from build123d import *

# Parameters (mm, degrees)
BOSS_EXTRU_1_DEPTH      = 18
ENL_V_MAT_EXTRU_1_REACH = 82.979
ESQUISSE4_W             = 11
ESQUISSE4_H             = 27
ENL_V_MAT_EXTRU_2_DEPTH = 11
D_GAGEMENT_M31_D        = 3.4
ENL_V_MAT_EXTRU_3_DEPTH = 8.4
ESQUISSE10_R            = 0.9
ENL_V_MAT_EXTRU_4_DEPTH = 4
ENL_V_MAT_EXTRU_5_DEPTH = 5
CONG_1_R                = 2
CONG_2_R                = 8
ENL_V_START             = -1.6
ESQUISSE13_R            = 1.5
ENL_V_MAT_EXTRU_6_DEPTH = 78.3514199


with BuildPart() as part:
    # Esquisse1 → Boss.-Extru.1 (new body)
    with BuildSketch(Plane(origin=(0, 0, 0), x_dir=(0, 0, -1), z_dir=(1, 0, 0))):
        Polygon((-37.5, 64.951905284), (-40.964101615, 62.951905284), (-24.964101615, 35.239092363), (-45.309401077, 0), (0, 0), (-2.309401077, 4), (-8.082903769, 4), (-23.232050808, 30.239092363), (-20.345299462, 35.239092363), align=None)
    extrude(amount=BOSS_EXTRU_1_DEPTH)

    # Esquisse4 → Enlèv. mat.-Extru.1 (cut, up to next)
    with BuildSketch(Plane(origin=(0, -2, 3.464101615), x_dir=(1, 0, 0), z_dir=(0, -0.5000000000000047, 0.8660254037844359)), mode=Mode.PRIVATE) as enl_v_mat_extru_1_sk1:
        with Locations((12.5, 61.5)):
            Rectangle(ESQUISSE4_W, ESQUISSE4_H)
    enl_v_mat_extru_1_tool1 = extrude(enl_v_mat_extru_1_sk1.sketch, amount=-ENL_V_MAT_EXTRU_1_REACH, mode=Mode.PRIVATE) & part.part
    add(enl_v_mat_extru_1_tool1.solids().sort_by_distance((12.5, 51.260562, 34.214102))[0], mode=Mode.SUBTRACT)

    # Esquisse6 → Enlèv. mat.-Extru.2 (cut)
    with BuildSketch(Plane(origin=(18, 0, 0), x_dir=(0, 0, -1), z_dir=(1, 0, 0))):
        Polygon((0, 0), (-2.309401077, 4), (-8.082903769, 4), (-5.773502692, 0), align=None)
    extrude(amount=-ENL_V_MAT_EXTRU_2_DEPTH, mode=Mode.SUBTRACT)

    # Dégagement M31 (through all)
    with Locations(Plane(origin=(0, 0, 0), x_dir=(-1, 0, 0), z_dir=(0, 0.5000000000000047, -0.866025403784436))):
        with Locations((-3.5, 71.2), (-3.5, 46)):
            Hole(D_GAGEMENT_M31_D / 2)

    # Esquisse9 → Enlèv. mat.-Extru.3 (cut)
    with BuildSketch(Plane.ZY):
        with BuildLine():
            Line((19.441451884, 15.2), (20.441451884, 16.2))
            Line((20.441451884, 16.2), (30.641451884, 16.2))
            Line((30.641451884, 16.2), (31.641451884, 15.2))
            Line((31.641451884, 15.2), (31.641451884, 13.4))
            ThreePointArc((31.641451884, 13.4), (32.541451884, 12.5), (31.641451884, 11.6))
            Line((31.641451884, 11.6), (31.641451884, 8.6))
            ThreePointArc((31.641451884, 8.6), (32.541451884, 7.7), (31.641451884, 6.8))
            Line((31.641451884, 6.8), (31.641451884, 5))
            Line((31.641451884, 5), (30.641451884, 4))
            Line((30.641451884, 4), (20.441451884, 4))
            Line((20.441451884, 4), (19.441451884, 5))
            Line((19.441451884, 5), (19.441451884, 6.8))
            ThreePointArc((19.441451884, 6.8), (18.541451884, 7.7), (19.441451884, 8.6))
            Line((19.441451884, 8.6), (19.441451884, 11.6))
            ThreePointArc((19.441451884, 11.6), (18.541451884, 12.5), (19.441451884, 13.4))
            Line((19.441451884, 13.4), (19.441451884, 15.2))
        make_face()
    extrude(amount=-ENL_V_MAT_EXTRU_3_DEPTH, mode=Mode.SUBTRACT)

    # Esquisse10 → Enlèv. mat.-Extru.4 (cut)
    with BuildSketch(Plane.ZY.offset(-8.4)):
        with Locations((19.441451884, 12.5)):
            Circle(ESQUISSE10_R)
        with Locations((19.441451884, 7.7)):
            Circle(ESQUISSE10_R)
        with Locations((31.641451884, 12.5)):
            Circle(ESQUISSE10_R)
        with Locations((31.641451884, 7.7)):
            Circle(ESQUISSE10_R)
    extrude(amount=-ENL_V_MAT_EXTRU_4_DEPTH, mode=Mode.SUBTRACT)

    # Esquisse11 → Enlèv. mat.-Extru.5 (cut)
    with BuildSketch(Plane.ZY):
        Polygon((25.541451884, 26.239092363), (12.701705922, 4), (38.381197846, 4), align=None)
    extrude(amount=-ENL_V_MAT_EXTRU_5_DEPTH, mode=Mode.SUBTRACT)

    # Congé1
    cong_1_edges = [part.edges().sort_by_distance(p)[0] for p in [
        (0, 63.951905284, 39.232050808),
        (2.5, 4, 38.381197846),
        (2.5, 26.239092363, 25.541451884),
        (2.5, 4, 12.701705922),
        (9, 0, 45.309401077),
        (9, 35.239092363, 24.964101615),
        (9, 35.239092363, 20.345299462),
        (9, 30.239092363, 23.232050808),
        (18, 40.569219382, 25.732050808),
        (7, 63.951905284, 39.232050808),
        (3.5, 0, 0),
        (3.5, 4, 8.082903769),
        (3.5, 4, 2.309401077),
        (12.5, 0, 5.773502692),
    ]]
    fillet(cong_1_edges, radius=CONG_1_R - 0.0001)  # a hair under: the kernel refuses the full size

    # Congé2
    cong_2_edges = [part.edges().sort_by_distance(p)[0] for p in [
        (7, 40.569219382, 25.732050808),
    ]]
    fillet(cong_2_edges, radius=CONG_2_R)

    # Esquisse13 → Enlèv. mat.-Extru.6 (cut, through all)
    with BuildSketch(Plane.ZY.offset(-8.4).offset(ENL_V_START)):
        with Locations((19.441451884, 12.5)):
            Circle(ESQUISSE13_R)
        with Locations((19.441451884, 7.7)):
            Circle(ESQUISSE13_R)
    extrude(amount=-ENL_V_MAT_EXTRU_6_DEPTH, mode=Mode.SUBTRACT)


solid = part.part
Read the model definition and answer for the solid it produces. Units are mm, in the model's axes. A direction names the side the tool comes from. Give positions to 0.01 mm unless a question says otherwise; leave off trailing zeros. Write each loop counter-clockwise with the first axis right and the second up, starting at its lowest first coordinate (ties: lowest second). Pieces come first, ordered by that corner, then holes. Notation, with made-up numbers: (-36, -40) - (-21, -40) arc R13 cw to (-21, -21) - close; hole circle Ø8 at (12.25, 18). An arc over 180 degrees is marked (long way). Answer in a Markdown table with one row per item. Add a question column.
Item 1: A tool of negligible diameter and unlimited length cuts with its end or side. For faces 1 (the face through (8.87, 32.72, 21.8)), 2 (the face through (6.87, 47.2, 27.25)), 3 (the face through (3, 4, 25)), 4 (the face through (9.28, 42.67, 26.91)), 5 (the face through (13.94, 7.13, 20.83)), from which of +Z, -Z, +X, -X, +Y, -Y can it reach the whole face along a straight path? Write none if from no direction.
Item 2: Section B-B, the plane z = 33.5 is taken. Write down the section's boundary in (x, y), and give its area (3 significant figures).
Item 3: Determine the mould class of faces 6 (the face through (7, 2, 5)), 7 (the face through (2.54, 24.24, 25.57)), 8 (the face through (3.549, 4.261, 7.915)) for opening direction Z: pulls with the +Z half, pulls with the -Z half, needs draft (parallel to the pull), parting line crosses it, or undercut.
Item 4: Find the intervals of material crossed by L1, parallel to Y at x = 1, z = 26; L2, parallel to Z at x = 8.8, y = 12.5; L3, parallel to Z at x = 8.85, y = 7.7, in increasing order.
Item 5: Flat-ended cylindrical pins translate along their axes: P1, Ø6, axis at y = 10.5, z = 25, coming from the -X side; P2, Ø2.5, axis at y = 13, z = 19.5, coming from the +X side; P3, Ø6, axis at y = 43.5, z = 29, coming from the +X side; P4, Ø10, axis at x = 10.5, y = 44, coming from the -Z side. Find the tip coordinate at first contact, or state that the pin passes through.
Item 6: Section D-D, the plane z = 15.5 is taken. Write down the section's boundary in (x, y).
Item 7: Section C-C, the plane x = 11.5 is taken. Write down the section's boundary in (y, z).
Item 8: Section A-A, the plane y = 12.5 is taken. Write down the section's boundary in (x, z), and give its area (3 significant figures).
Recorded:
| question | item | result |
|---|---|---|
| 1 | face 1 | -Z, +X, -X |
| 1 | face 2 | -Z, +X, -X, +Y |
| 1 | face 3 | -X |
| 1 | face 4 | +Z, +X, +Y |
| 1 | face 5 | +X |
| 2 | outline | (0, 0) - (18, 0) - (18, 20.45) - (0, 20.45) - (0, 12.45) - (5, 12.45) - (5, 4) - (0, 4) - close; (0, 50.02) - (7, 50.02) - (7, 58.02) - (0, 58.02) - close |
| 2 | area | 382 mm2 |
| 3 | face 6 | needs draft |
| 3 | face 7 | undercut |
| 3 | face 8 | pulls with the -Z half |
| 4 | L1 | y = 0 to 4, 24.19 to 33.44, 37.03 to 45.03 |
| 4 | L2 | z = 12.99 to 18.54, 20.34 to 30.74, 32.54 to 38.09 |
| 4 | L3 | z = 10.22 to 18.54, 20.34 to 30.74, 32.54 to 40.86 |
| 5 | P1 | stops at x = 8.4 |
| 5 | P2 | stops at x = 18 |
| 5 | P3 | stops at x = 10.83 |
| 5 | P4 | stops at z = 22.52 |
| 6 | outline | (0, 0) - (18, 0) - (18, 16.85) - (0, 16.85) - (0, 8.85) - (5, 8.85) - (5, 4.11) - (0, 4.11) - close |
| 7 | outline | (0, 9.24) arc R2 ccw to (3, 7.51) - (29.24, 22.65) arc R2 cw to (31.24, 22.65) - (34.24, 20.92) arc R2 ccw to (36.24, 20.92) - (42.27, 24.4) - (40.27, 27.87) - (36.24, 25.54) arc R2 cw to (34.24, 25.54) - (3, 43.58) arc R2 ccw to (0, 41.85) - close; hole circle Ø3 at (7.7, 19.44); hole circle Ø1.8 at (7.7, 31.64); hole circle Ø3 at (12.5, 19.44); hole circle Ø1.8 at (12.5, 31.64) |
| 8 | outline | (0, 12.99) - (18, 12.99) - (18, 17.94) - (10, 17.94) - (10, 18.54) - (5, 18.54) - (5, 17.61) - (0, 17.61) - close; (0, 33.47) - (5, 33.47) - (5, 32.54) - (12.4, 32.54) - (12.4, 30.74) - (8.4, 30.74) - (8.4, 20.34) - (10, 20.34) - (10, 20.94) - (18, 20.94) - (18, 38.09) - (0, 38.09) - close |
| 8 | area | 291 mm2 |
